from build123d import *

# Parameters (mm, degrees)
SKETCH1_W                = 203.2
SKETCH1_H                = 254.254
SKETCH1_W_2              = 138.43
SKETCH1_H_2              = 228.9175
BOSS_EXTRUDE1_DEPTH      = 1.5875
BOSS_EXTRUDE1_DEPTH_BACK = 12.7
SKETCH2_W                = 10.16
SKETCH2_H                = 12.7
BOSS_EXTRUDE2_DEPTH      = 10.16
SKETCH3_W                = 15.24
SKETCH3_H                = 29.693732077
BOSS_EXTRUDE3_DEPTH      = 6.578885717
SKETCH5_W                = 6.578885717
SKETCH5_H                = 29.693732077
BOSS_EXTRUDE4_DEPTH      = 26.162
SKETCH6_R                = 6.604
BOSS_EXTRUDE6_DEPTH      = 76.2
SKETCH11_R               = 6.604
CUT_EXTRUDE3_DEPTH       = 5.842
SKETCH13_R               = 5.4991
BOSS_EXTRUDE7_DEPTH      = 5.842
SKETCH15_W               = 15.24
SKETCH15_H               = 29.693732077
BOSS_EXTRUDE8_DEPTH      = 50.8
SKETCH16_W               = 14.2875
SKETCH16_H               = 112.267770999
BOSS_EXTRUDE9_DEPTH      = 57.15
SKETCH17_W               = 14.2875
SKETCH17_H               = 112.292496924
BOSS_EXTRUDE10_DEPTH     = 57.658
SKETCH18_R               = 7.9375
CUT_EXTRUDE4_DEPTH       = 57.658


with BuildPart() as part:
    # Sketch1 → Boss-Extrude1 (new body, two sides)
    with BuildSketch(Plane.XY) as boss_extrude1_sk:
        with Locations((18.415, 0)):
            Rectangle(SKETCH1_W, SKETCH1_H)
        Rectangle(SKETCH1_W_2, SKETCH1_H_2, mode=Mode.SUBTRACT)
    extrude(amount=BOSS_EXTRUDE1_DEPTH)
    extrude(boss_extrude1_sk.sketch, amount=-BOSS_EXTRUDE1_DEPTH_BACK)

    # Sketch2 → Boss-Extrude2 (add)
    with BuildSketch(Plane.XY.offset(1.5875)):
        with Locations((-76.2, 0)):
            Rectangle(SKETCH2_W, SKETCH2_H)
    extrude(amount=BOSS_EXTRUDE2_DEPTH)

    # Sketch3 → Boss-Extrude3 (add)
    with BuildSketch(Plane.ZY.offset(83.185)):
        with Locations((-6.0325, 0.012362963)):
            Rectangle(SKETCH3_W, SKETCH3_H)
    extrude(amount=BOSS_EXTRUDE3_DEPTH)

    # Sketch5 → Boss-Extrude4 (add)
    with BuildSketch(Plane.XY.offset(1.5875)):
        with Locations((-86.474442858, 0.012362963)):
            Rectangle(SKETCH5_W, SKETCH5_H)
    extrude(amount=BOSS_EXTRUDE4_DEPTH)

    # Sketch6 → Boss-Extrude6 (add)
    with BuildSketch(Plane(origin=(-83.185, 0, 0), x_dir=(0, 0, -1), z_dir=(1, 0, 0))):
        with Locations((-19.291204972, 0)):
            Circle(SKETCH6_R)
    extrude(amount=-BOSS_EXTRUDE6_DEPTH)

    # Sketch11 → Cut-Extrude3 (cut)
    with BuildSketch(Plane(origin=(-83.185, 0, 0), x_dir=(0, 0, -1), z_dir=(1, 0, 0))):
        with Locations((-19.291204972, 0)):
            Circle(SKETCH11_R)
    extrude(amount=-CUT_EXTRUDE3_DEPTH, mode=Mode.SUBTRACT)

    # Sketch13 → Boss-Extrude7 (add)
    with BuildSketch(Plane(origin=(-89.027, 0, 0), x_dir=(0, 0, -1), z_dir=(1, 0, 0))):
        with Locations((-19.291204972, 0)):
            Circle(SKETCH13_R)
    extrude(amount=BOSS_EXTRUDE7_DEPTH)

    # Sketch15 → Boss-Extrude8 (add)
    with BuildSketch(Plane.ZY.offset(89.763885717)):
        with Locations((-6.0325, 0.012362963)):
            Rectangle(SKETCH15_W, SKETCH15_H)
    extrude(amount=BOSS_EXTRUDE8_DEPTH)

    # Sketch16 → Boss-Extrude9 (add)
    with BuildSketch(Plane.ZY.offset(83.185)):
        with Locations((-5.55625, 70.9931145)):
            Rectangle(SKETCH16_W, SKETCH16_H)
    extrude(amount=BOSS_EXTRUDE9_DEPTH)

    # Sketch17 → Boss-Extrude10 (add)
    with BuildSketch(Plane.ZY.offset(83.185)):
        with Locations((-5.55625, -70.980751538)):
            Rectangle(SKETCH17_W, SKETCH17_H)
    extrude(amount=BOSS_EXTRUDE10_DEPTH)

    # Sketch18 → Cut-Extrude4 (cut)
    with BuildSketch(Plane.XY.offset(1.5875)):
        with Locations((-93.141229835, 58.590088082)):
            Circle(SKETCH18_R)
    extrude(amount=-CUT_EXTRUDE4_DEPTH, mode=Mode.SUBTRACT)


solid = part.part
CAD build for the part. Positions are in the model's coordinates, mm. A direction names the side the tool comes from. Give positions to 0.01 mm unless a question says otherwise; leave off trailing zeros. Write each loop counter-clockwise with the first axis right and the second up, starting at its lowest first coordinate (ties: lowest second). Pieces come first, ordered by that corner, then holes. Notation, with made-up numbers: (17, 30.25) -> (52, 30.25) arc R17 ccw to (52, 39.25) -> close; hole circle Ø4 at (1, 49.5). An arc over 180 degrees is marked (long way). Return JSON: item names as keys, results as strings.
Item 1: Drill centre lines: probe 1 along Y at (x, z) = (-11, -4.5); probe 2 along X at (y, z) = (16, -8) (3 decimals); probe 3 along X at (y, z) = (-5.5, -2) (3 decimals). Where is each one in solid material? Low to high.
Answer below:
{"probe 1": "y = -127.13 to -114.46, 114.46 to 127.13", "probe 2": "x = -140.335 to -69.215, 69.215 to 120.015", "probe 3": "x = -140.564 to -69.215, 69.215 to 120.015"}
Item 2: Tool access for faces 1 (the flat face through (-140.335, 72, -6)), 2 (the flat face through (-89.764, 0, 12)), 3 (the flat face through (-76, 6.35, 7)): list every direction of +Z, -Z, +X, -X, +Y, -Y with a clear straight run to the whole face (end or side of a thin tool).
Answer below:
{"face 1": "+Z, -Z, -X, +Y", "face 2": "-X", "face 3": "+Z, +X, +Y"}
Item 3: Drop flat-ended pins along their axis: pin 1 (5.5 mm diameter, centred on x = -85, z = 13, fed in from -Y); pin 2 (15.5 mm diameter, centred on y = 58.5, z = -6, fed in from -X) (3 decimals); pin 3 (3 mm diameter, centred on y = 1, z = 7.5, fed in from +X); pin 4 (8 mm diameter, centred on x = -26.5, z = 6, fed in from -Y). Give the stop position or say it passes through.
Answer below:
{"pin 1": "stops at y = -14.83", "pin 2": "stops at x = -140.335", "pin 3": "stops at x = -71.12", "pin 4": "passes through"}
Item 4: Two-plate mould, pull along Y, no slides. Class faces 4 (the flat face through (69.215, -2, -5)), 5 (the flat face through (-8, 127.127, -6)), 6 (the flat face through (-140.564, 0, -6)): +Y half, -Y half, draft (parallel to the pull), parting line (faces both ways), or undercut.
Answer below:
{"face 4": "undercut", "face 5": "+Y half", "face 6": "draft"}
Item 5: Band-saw the part on C-C (x = -45.5). List the corners of the cut face in (y, z), then the cut area to 3 significant figures.
Answer below:
{"outline": "(-127.13, -12.7) -> (-114.46, -12.7) -> (-114.46, 1.59) -> (-127.13, 1.59) -> close; (114.46, -12.7) -> (127.13, -12.7) -> (127.13, 1.59) -> (114.46, 1.59) -> close", "area": "362 mm2"}
